```python
from build123d import *

# Parameters (mm, degrees)
SKETCH2_R           = 5.08
SKETCH2_R_2         = 3.175
BOSS_EXTRUDE1_DEPTH = 19.05
CUT_EXTRUDE1_DEPTH  = 12.7
CUT_EXTRUDE2_DEPTH  = 6.35


with BuildPart() as part:
    # Sketch2 → Boss-Extrude1 (new body)
    with BuildSketch(Plane(origin=(0, 0, 0), x_dir=(0, 0, -1), z_dir=(1, 0, 0))):
        with BuildLine():
            Line((-270.378794472, -38.1), (270.378794472, -38.1))
            ThreePointArc((270.378794472, -38.1), (273.05, 0), (270.378794472, 38.1))
            Line((270.378794472, 38.1), (38.1, 38.1))
            Line((38.1, 38.1), (-270.378794472, 38.1))
            ThreePointArc((-270.378794472, 38.1), (-273.05, 0), (-270.378794472, -38.1))
        make_face()
        with Locations(Location((249.2375, 0, 0), (0, 0, 180))):
            Circle(SKETCH2_R, mode=Mode.SUBTRACT)
        with Locations(Location((261.240141142, -19.100852393, 0), (0, 0, 180))):
            Circle(SKETCH2_R_2, mode=Mode.SUBTRACT)
        with Locations(Location((-261.240141142, -19.100852393, 0), (0, 0, 180))):
            Circle(SKETCH2_R_2, mode=Mode.SUBTRACT)
        with Locations(Location((-238.949490115, -19.110830171, 0), (0, 0, 180))):
            Circle(SKETCH2_R_2, mode=Mode.SUBTRACT)
        with Locations(Location((-217.4875, 0, 0), (0, 0, 180))):
            Circle(SKETCH2_R, mode=Mode.SUBTRACT)
        with Locations(Location((-153.9875, 0, 0), (0, 0, 180))):
            Circle(SKETCH2_R, mode=Mode.SUBTRACT)
        with Locations(Location((-90.4875, 0, 0), (0, 0, 180))):
            Circle(SKETCH2_R, mode=Mode.SUBTRACT)
        with Locations(Location((-19.05, 0, 0), (0, 0, 180))):
            Circle(SKETCH2_R_2, mode=Mode.SUBTRACT)
        with Locations(Location((0, -19.05, 0), (0, 0, 180))):
            Circle(SKETCH2_R_2, mode=Mode.SUBTRACT)
        with Locations(Location((238.949490115, -19.110830171, 0), (0, 0, 180))):
            Circle(SKETCH2_R_2, mode=Mode.SUBTRACT)
        with Locations(Location((19.05, 0, 0), (0, 0, 180))):
            Circle(SKETCH2_R_2, mode=Mode.SUBTRACT)
        with Locations(Location((58.7375, 0, 0), (0, 0, 180))):
            Circle(SKETCH2_R, mode=Mode.SUBTRACT)
        with Locations(Location((122.2375, 0, 0), (0, 0, 180))):
            Circle(SKETCH2_R, mode=Mode.SUBTRACT)
        with Locations(Location((185.7375, 0, 0), (0, 0, 180))):
            Circle(SKETCH2_R, mode=Mode.SUBTRACT)
        with Locations(Location((-261.240141142, 19.100852393, 0), (0, 0, 180))):
            Circle(SKETCH2_R_2, mode=Mode.SUBTRACT)
        with Locations(Location((-238.949490115, 19.110830171, 0), (0, 0, 180))):
            Circle(SKETCH2_R_2, mode=Mode.SUBTRACT)
        with Locations(Location((0, 19.05, 0), (0, 0, 180))):
            Circle(SKETCH2_R_2, mode=Mode.SUBTRACT)
        with Locations(Location((238.949490115, 19.110830171, 0), (0, 0, 180))):
            Circle(SKETCH2_R_2, mode=Mode.SUBTRACT)
        with Locations(Location((261.240141142, 19.100852393, 0), (0, 0, 180))):
            Circle(SKETCH2_R_2, mode=Mode.SUBTRACT)
    extrude(amount=BOSS_EXTRUDE1_DEPTH)

    # Sketch3 → Cut-Extrude1 (cut)
    with BuildSketch(Plane(origin=(19.05, 0, 0), x_dir=(0, 0, -1), z_dir=(1, 0, 0))):
        Polygon((21.997045256, -38.1), (65.991135768, 38.1), (-21.997045256, 38.1), (-65.991135768, -38.1), align=None)
    extrude(amount=-CUT_EXTRUDE1_DEPTH, mode=Mode.SUBTRACT)

    # Sketch3_3 → Cut-Extrude2 (cut)
    with BuildSketch(Plane(origin=(19.05, 0, 0), x_dir=(0, 0, -1), z_dir=(1, 0, 0))):
        Polygon((-43.994090512, 0), (-38.1, 10.208864232), (-38.1, 38.1), (-65.991135768, 38.1), align=None)
        Polygon((-38.1, 38.1), (-38.1, 10.208864232), (-21.997045256, 38.1), align=None)
        Polygon((21.997045256, -38.1), (38.1, -38.1), (38.1, -10.208864232), align=None)
        Polygon((38.1, -10.208864232), (38.1, -38.1), (65.991135768, -38.1), (43.994090512, 0), align=None)
    extrude(amount=-CUT_EXTRUDE2_DEPTH, mode=Mode.SUBTRACT)


solid = part.part
```
Check sheet for the modelled part. Datum: model origin and axes. Units: mm. A direction names the side the tool comes from. Coordinates: 2 decimals unless noted, no trailing zeros. Write each loop counter-clockwise with the first axis right and the second up, starting at its lowest first coordinate (ties: lowest second). Pieces come first, ordered by that corner, then holes. Notation, with made-up numbers: M -40,71 L -10,71 A21 cw -10,88 Z; hole C 24,68.5 d8. An arc over 180 degrees is marked long. Use one line per item in the form item = value.
Item 1: Release check for a two-part mould opening along Z. For faces 1 (the face through (9.392, 1.946, -181.045)), 2 (the face through (9.39, -0.54, -273.05)), 3 (the face through (0, 1, 4)) record: pulls with the +Z half, pulls with the -Z half, needs draft (parallel to the pull), parting line crosses it, or undercut.
Answer below:
face_1 = undercut
face_2 = pulls with the -Z half
face_3 = needs draft
Item 2: Sectioned sample at A-A, the plane z = -27. Record the cut outline in (x, y), and give its area (3 significant figures).
Answer below:
outline = M 0,-38.1 L 12.7,-38.1 L 12.7,-29.43 L 6.35,-29.43 L 6.35,38.1 L 0,38.1 Z
area = 539 mm^2
Item 3: Material ranges on L1, parallel to Z at x = 9.75, y = -18; L2, parallel to Z at x = 15.5, y = 33; L3, parallel to X at y = -28, z = 48, recorded low to high. Write a range as from..to.
Answer below:
L1 = -272.46..-264.22, -258.26..-241.92, -235.98..-33.6, 54.39..235.98, 241.92..258.26, 264.22..272.46
L2 = -271.05..-63.05, 63.05..271.05
L3 = 0..6.35
Item 4: Gauge pin test, flat ends, axial feed: pin 1 Ø1 at (x, y) = (8, -21.5) entering from -Z; pin 2 Ø19 at (y, z) = (-19, -34) entering from +X; pin 3 Ø5.5 at (y, z) = (-19.05, 0) entering from +X; pin 4 Ø6 at (x, z) = (17, -52.5) entering from +Y. Record the tip position at first contact, or that the pin passes through.
Answer below:
pin_1 = -272.24
pin_2 = 12.7
pin_3 = through
pin_4 = 19.93
Item 5: Set-up check for faces 4 (the face through (9.392, -0.223, 148.912)), 5 (the face through (6.35, 1, 1)), 6 (the face through (11.378, 7.933, -48.574)), 7 (the face through (11.378, -7.933, 48.574)): record each of +Z, -Z, +X, -X, +Y, -Y from which the full face is reachable in a straight line by a thin tool's end or side.
Answer below:
face_4 = +X, -X
face_5 = +X
face_6 = +X, +Y
face_7 = +X, -Y
